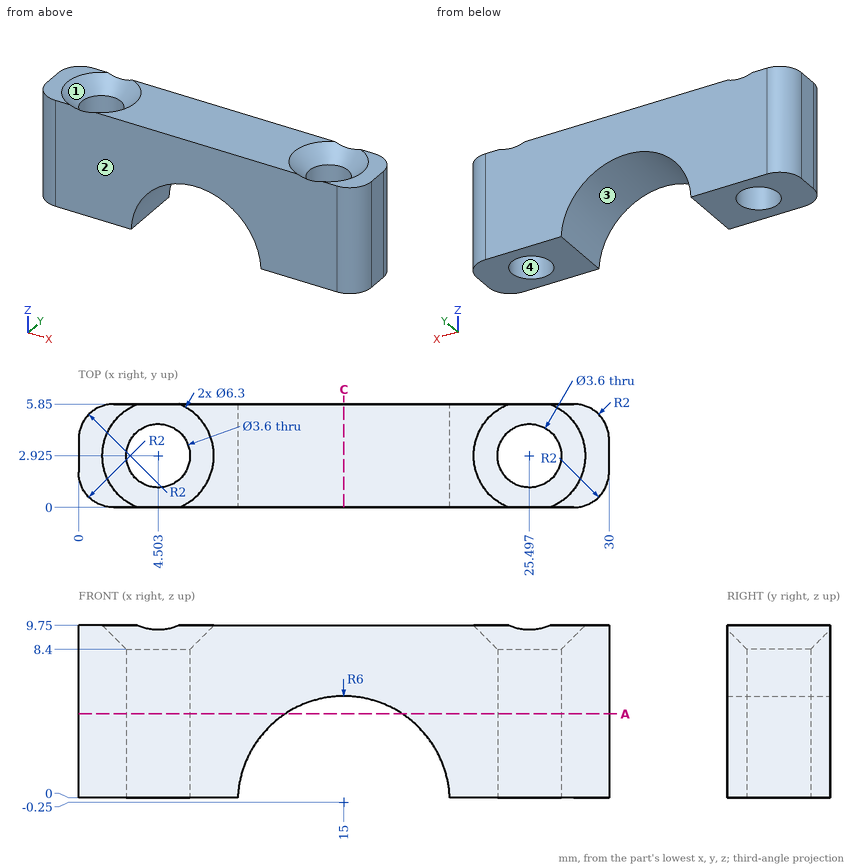
The figure shows three views and two pictorial views of one solid part (mm, origin at its lowest corner). Answer the questions. Coordinates: 2 decimals unless noted, no trailing zeros. Order: outer loops, then holes, each group sorted by start corner. A loop starts at its lowest first (then second) coordinate and runs counter-clockwise, first axis right, second up.
Q1. For a pull along Y with two mould halves and no side action, classify the marked faces 1, 2, 3 and 4 as pulls with the +Y half, pulls with the -Y half, needs draft (parallel to the pull), parting line crosses it, or undercut.
Q2. Given P1, Ø1, axis at x = 4.5, y = 3.5, coming from the -Z side, flat-ended and moving along its own axis, determine where the tip first touches the part or whether it passes through.
Q3. A cutting plane is placed at A-A, the plane z = 4.75. State how many separate pieces and enclosed holes the cut face has, and give its area (3 significant figures).
Q4. Consider line 1 (X direction, y = 2.4, z = 7) (1 decimal); line 2 (X direction, y = 3.3, z = 4) (1 decimal); line 3 (X direction, y = 4.6, z = 9) (1 decimal). Determine where each line is inside the solid, lowest interval first.
Q5. A cutting plane is placed at C-C, the plane x = 15. Write down the section's boundary in (y, z), and give its area (3 significant figures).
Answers follow:
1. face 1: undercut
1. face 2: pulls with the -Y half
1. face 3: needs draft
1. face 4: undercut
2. P1: passes through
3. separate pieces: 2
3. enclosed holes: 2
3. area: 113 mm2
4. line 1: x = 0 to 2.8, 6.2 to 23.8, 27.2 to 30
4. line 2: x = 0 to 2.7, 6.3 to 10.8, 19.2 to 23.7, 27.3 to 30
4. line 3: x = 0.1 to 2.8, 6.2 to 23.8, 27.2 to 29.9
5. outline: (0, 5.75) - (5.85, 5.75) - (5.85, 9.75) - (0, 9.75) - close
5. area: 23.4 mm2
